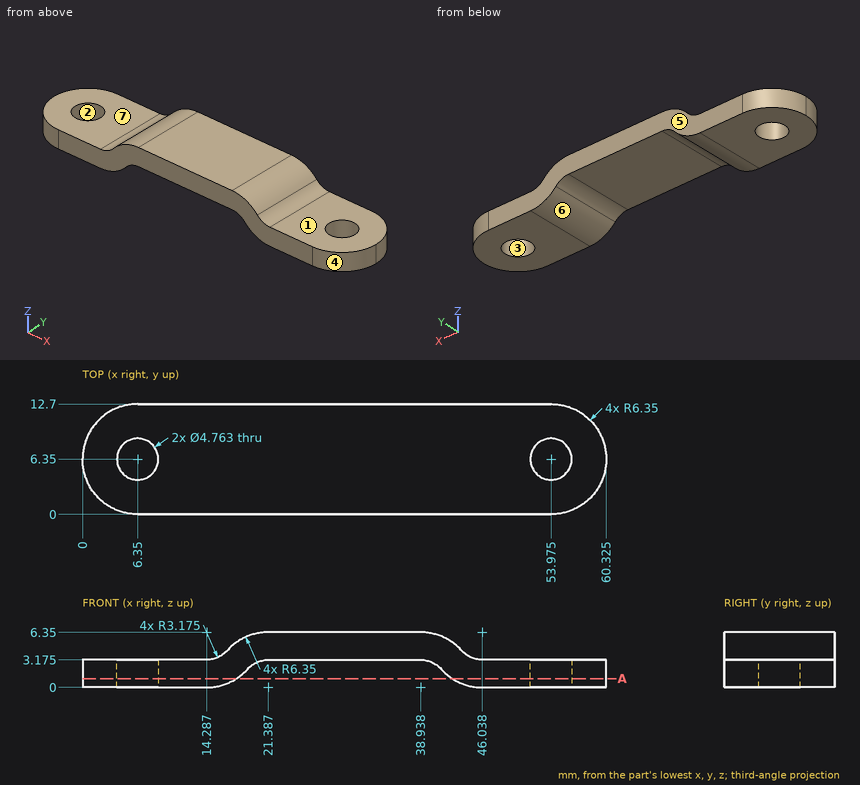
Study the drawing (mm; zero at the part's minimum x, y, z) and answer. A direction names the side the tool comes from. Give positions to 0.01 mm unless a question says otherwise; leave off trailing zeros. Answer as CSV lines item,"result". Start each with the question number.
1) Which of the six approach directions +Z, -Z, +X, -X, +Y, -Y give full straight-line access (tool end or side, diameter ignored) to the marked faces 5, 6 and 7?
2) Find section A-A (z = 1). State how many separate pieces and enclosed holes the cut face has.
3) Determine the mould class of the marked faces 1, 2, 3 and 4 for opening direction Y: released by +Y, released by -Y, zero draft, split by the parting line, or undercut.
4) Straight lines are drawn through the part: L1, parallel to X at y = 7, z = 0.5 (1 decimal); L2, parallel to Z at x = 13, y = 10 (1 decimal); L3, parallel to X at y = 1, z = 1 (1 decimal). For each, find the intervals that lie inside material, in ascending order. Write a range as from..to.
5) Each of these flat-tipped pins is pushed along its axis until it touches: pin 1 Ø2 at (y, z) = (7.5, 3.5) entering from +X; pin 2 Ø3 at (y, z) = (8.5, 5.5) entering from -X; pin 3 Ø1.5 at (y, z) = (9.5, 3.5) entering from +X. Where does it stop, or does it pass through?
Findings below:
1,face 5,"+Z, -Z, +X, -X, +Y"
1,face 6,"-Z, +Y, -Y"
1,face 7,"+Z, -X, +Y, -Y"
2,separate pieces,"2"
2,enclosed holes,"2"
3,face 1,"zero draft"
3,face 2,"undercut"
3,face 3,"undercut"
3,face 4,"released by -Y"
4,L1,"0..4.1, 8.6..16.8, 43.6..51.7, 56.3..60.3"
4,L2,"0..3.2"
4,L3,"2.9..17.7, 42.6..57.4"
5,pin 1,"x = 60.32"
5,pin 2,"x = 16.42"
5,pin 3,"x = 59.82"
